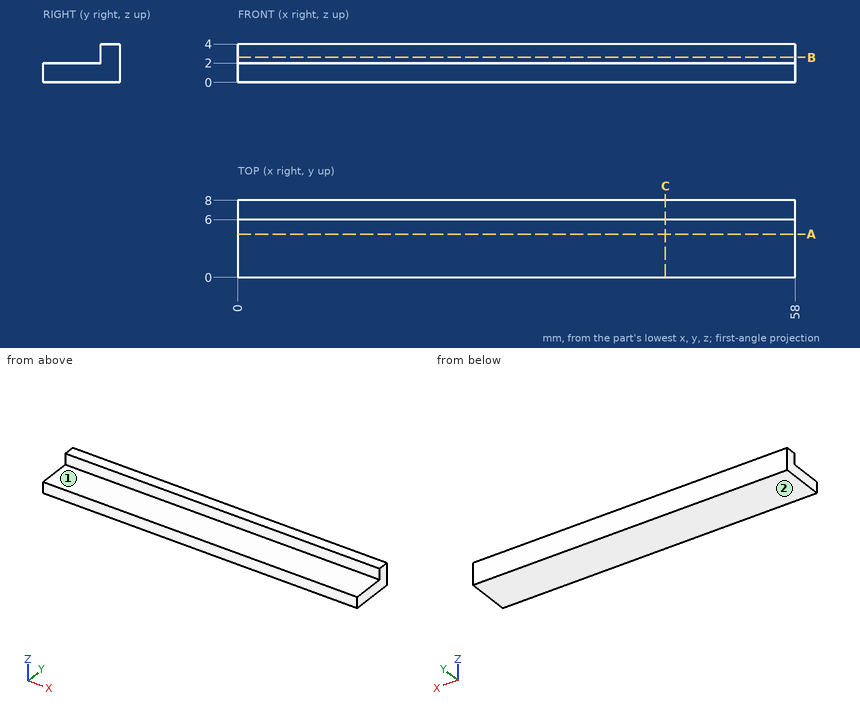
Drawing for the job (mm, zero at the part's lowest x, y, z). A direction names the side the tool comes from. Round coordinates to 2 decimals unless told otherwise and drop trailing zeros. Order: outer loops, then holes, each group sorted by start corner. A loop starts at its lowest first (then second) coordinate and runs counter-clockwise, first axis right, second up. Notation, with made-up numbers: (23, 51.5) -> (64, 51.5) arc R16 cw to (64, 64.5) -> close; hole circle Ø4 at (-3.5, 19.25). An arc over 180 degrees is marked (long way). Write item = value, one per line. Start each with the question number.
(1) Cut at C-C, the plane x = 44.5. List the corners of the cut face in (y, z).
(2) Probe line 1 (Z direction, x = 33, y = 3.5); line 2 (Y direction, x = 44.5, z = 2.25). List the from-to ranges inside material, lowest first. Write a range as [from, to].
(3) Pin check, flat tips, straight feed: P1, Ø1.6, axis at x = 18, z = 3, coming from the -Y side; P2, Ø3, axis at x = 47, y = 2.5, coming from the +Z side; P3, Ø1, axis at x = 15.5, z = 1, coming from the -Y side. Stop position of each tip, or through.
(4) Cut at B-B, the plane z = 2.6. List the corners of the cut face in (x, y).
(5) Which spindle directions (+Z, -Z, +X, -X, +Y, -Y) get a long thin tool onto all of the face, cutting with end or side? Do the marked faces 1 and 2. Say none if no direction does.
(6) Cut at A-A, the plane y = 4.5. List the corners of the cut face in (x, z), then the cut area to 3 significant figures.
Model answer:
q1.outline = (0, 0) -> (8, 0) -> (8, 4) -> (6, 4) -> (6, 2) -> (0, 2) -> close
q2.line_1 = [0, 2]
q2.line_2 = [6, 8]
q3.P1 = 6
q3.P2 = 2
q3.P3 = 0
q4.outline = (0, 6) -> (58, 6) -> (58, 8) -> (0, 8) -> close
q5.face_1 = +Z, +X, -X, -Y
q5.face_2 = -Z, +X, -X, +Y, -Y
q6.outline = (0, 0) -> (58, 0) -> (58, 2) -> (0, 2) -> close
q6.area = 116 mm2
